```python
from build123d import *

# Parameters (mm, degrees)
SKETCH_1_W      = 500
SKETCH_1_H      = 500
EXTRUDE_1_DEPTH = 50
SKETCH_2_W      = 50
SKETCH_2_H      = 50
EXTRUDE_2_DEPTH = 450
SKETCH_3_W      = 50
SKETCH_3_H      = 50
EXTRUDE_3_DEPTH = 450
SKETCH_4_W      = 50
SKETCH_4_H      = 50
EXTRUDE_4_DEPTH = 450
SKETCH_5_W      = 50
SKETCH_5_H      = 50
EXTRUDE_5_DEPTH = 450
SKETCH_6_W      = 400
SKETCH_6_H      = 50
EXTRUDE_6_DEPTH = 400
SKETCH_7_W      = 50
SKETCH_7_H      = 300
EXTRUDE_7_DEPTH = 150
SKETCH_8_W      = 50
SKETCH_8_H      = 300
EXTRUDE_8_DEPTH = 150


with BuildPart() as part:
    # 草图1 → 凸台-拉伸1 (new body)
    with BuildSketch(Plane.XY):
        Rectangle(SKETCH_1_W, SKETCH_1_H)
    extrude(amount=EXTRUDE_1_DEPTH)

    # 草图2 → 凸台-拉伸2 (add)
    with BuildSketch(Plane.XY):
        with Locations((-200, -200)):
            Rectangle(SKETCH_2_W, SKETCH_2_H)
    extrude(amount=EXTRUDE_2_DEPTH)

    # 草图3 → 凸台-拉伸3 (add)
    with BuildSketch(Plane.XY):
        with Locations((200, -200)):
            Rectangle(SKETCH_3_W, SKETCH_3_H)
    extrude(amount=EXTRUDE_3_DEPTH)

    # 草图4 → 凸台-拉伸4 (add)
    with BuildSketch(Plane.XY):
        with Locations((-200, 200)):
            Rectangle(SKETCH_4_W, SKETCH_4_H)
    extrude(amount=EXTRUDE_4_DEPTH)

    # 草图5 → 凸台-拉伸5 (add)
    with BuildSketch(Plane.XY):
        with Locations((200, 200)):
            Rectangle(SKETCH_5_W, SKETCH_5_H)
    extrude(amount=EXTRUDE_5_DEPTH)

    # 草图6 → 凸台-拉伸6 (add)
    with BuildSketch(Plane(origin=(0, 0, 0), x_dir=(-1, 0, 0), z_dir=(0, 0, -1))):
        Rectangle(SKETCH_6_W, SKETCH_6_H)
    extrude(amount=EXTRUDE_6_DEPTH)

    # 草图7 → 凸台-拉伸7 (add)
    with BuildSketch(Plane(origin=(225, 0, 0), x_dir=(0, 0, -1), z_dir=(1, 0, 0))):
        with Locations((0, 200)):
            Rectangle(SKETCH_7_W, SKETCH_7_H)
    extrude(amount=EXTRUDE_7_DEPTH)

    # 草图8 → 凸台-拉伸8 (add)
    with BuildSketch(Plane.ZY.offset(225)):
        with Locations((0, 200)):
            Rectangle(SKETCH_8_W, SKETCH_8_H)
    extrude(amount=EXTRUDE_8_DEPTH)


solid = part.part
```
Geometry: final body of the model. Coordinates: model frame, mm. A direction names the side the tool comes from. Round coordinates to 2 decimals unless told otherwise and drop trailing zeros. Order: outer loops, then holes, each group sorted by start corner. A loop starts at its lowest first (then second) coordinate and runs counter-clockwise, first axis right, second up. Notation, with made-up numbers: M -26.75,-14.75 L 1.25,-14.75 A17 ccw 1.25,-9.75 Z; hole C -4.5,79.5 d3. An arc over 180 degrees is marked long. Use one line per item in the form item = value. Start each with the question number.
Q1. Pin query (flat end, axial travel): pin 1 Ø25 at (y, z) = (207.5, 240.5) entering from +X; pin 2 Ø5 at (x, y) = (-74.5, 127) entering from +Z; pin 3 Ø15 at (x, z) = (202, 326) entering from +Y. Return the tip coordinate at first contact, or that it passes through.
Q2. Mould query, pull axis Y, two halves, no side actions, for faces 6 (the face through (200, 175, 247)), 7 (the face through (299, 350, 0)), 8 (the face through (-200, -175, 247)), 9 (the face through (-175, -200, 247)). Classes: +Y half, -Y half, draft (parallel to the pull), parting line (faces both ways), or undercut.
Q3. Cut plane B-B (z = 221.5). Return loops of the section in (x, y).
Q4. Access query for faces 1 (the face through (3, 25, -197)), 2 (the face through (-200, 225, 247)), 3 (the face through (-225, 235, -6)), 4 (the face through (175, 200, 247)), 5 (the face through (200, 0, -197)). Directions: +Z, -Z, +X, -X, +Y, -Y. A direction counts if a zero-diameter tool reaches every point of the face in a straight line with its end or side. Return the directions, or none.
Q5. Cut plane D-D (x = 102.5). Return loops of the section in (y, z).
Q6. Material intervals for line 1 (X direction, y = -193, z = 241); line 2 (Z direction, x = -76.5, y = 209), sorted ascending. Write a range as [from, to].
Q7. Cut plane A-A (y = 277.5). Return loops of the section in (x, z).
Q8. Cut plane C-C (y = 89). Return loops of the section in (x, z), and give its area (4 significant figures).
Geometry results:
q1.pin_1 = 225
q1.pin_2 = 50
q1.pin_3 = 225
q2.face_6 = undercut
q2.face_7 = +Y half
q2.face_8 = undercut
q2.face_9 = draft
q3.outline = M -225,-225 L -175,-225 L -175,-175 L -225,-175 Z; M -225,175 L -175,175 L -175,225 L -225,225 Z; M 175,-225 L 225,-225 L 225,-175 L 175,-175 Z; M 175,175 L 225,175 L 225,225 L 175,225 Z
q4.face_1 = -Z, +X, -X, +Y
q4.face_2 = +Z, +X, -X, +Y
q4.face_3 = -Z, +Y
q4.face_4 = +Z, +Y, -Y
q4.face_5 = -Z, +X, +Y, -Y
q5.outline = M -250,0 L -25,0 L -25,-400 L 25,-400 L 25,0 L 250,0 L 250,50 L -250,50 Z
q6.line_1 = [-225, -175], [175, 225]
q6.line_2 = [0, 50]
q7.outline = M -375,-25 L -225,-25 L -225,25 L -375,25 Z; M 225,-25 L 375,-25 L 375,25 L 225,25 Z
q8.outline = M -375,-25 L -225,-25 L -225,0 L 225,0 L 225,-25 L 375,-25 L 375,25 L 250,25 L 250,50 L -250,50 L -250,25 L -375,25 Z
q8.area = 38,750 mm^2
